Input: part model. Units: mm. Frame: model coordinates. Face numbers are marked on the shaded views. A direction names the side the tool comes from. Coordinates: 2 decimals unless noted, no trailing zeros. Order: outer loops, then holes, each group sorted by start corner. A loop starts at its lowest first (then second) coordinate and runs counter-clockwise, first axis right, second up. Notation, with made-up numbers: (0, -8.75) - (46, -8.75) arc R20 ccw to (46, 3.25) - close; hole circle Ø2 at (29, 5.5). An arc over 180 degrees is marked (long way). Answer as CSV lines item,"result". Start each with the question number.
Item 1: Draft query along Y for the marked faces 1, 2 and 3. Return one class per face: +Y half, -Y half, draft (parallel to the pull), parting line (faces both ways), or undercut.
Item 2: First-contact query: pin 1 (6 mm diameter, centred on x = -12, y = 4.5, fed in from -Z); pin 2 (11 mm diameter, centred on x = -1.5, z = 37.5, fed in from +Y); pin 3 (1 mm diameter, centred on x = 11.5, z = 77, fed in from +Y). Flat tips, straight axial feed; report the tip coordinate or a pass-through.
Item 3: Section D-D (x = 17). Output: boundary loops of the cut face in (y, z), and give its area (3 significant figures).
Item 4: Access query for the marked faces 4 and 5. Directions: +Z, -Z, +X, -X, +Y, -Y. A direction counts if a zero-diameter tool reaches every point of the face in a straight line with its end or side. Return the directions, or none.
Item 5: Material intervals for line 1 along Z through (x, y) = (0, -14); line 2 along X through (y, z) = (3, 63.5); line 3 along Y through (x, z) = (-1, 41.5), sorted ascending.
Item 6: Section A-A (x = 0). Output: boundary loops of the cut face in (y, z), and give its area (3 significant figures).
Item 7: Section C-C (y = 8.5). Output: boundary loops of the cut face in (x, z), and give its area (3 significant figures).
Item 8: Section B-B (z = 83.5). Output: boundary loops of the cut face in (x, y) (1 decimal), and give its area (3 significant figures).
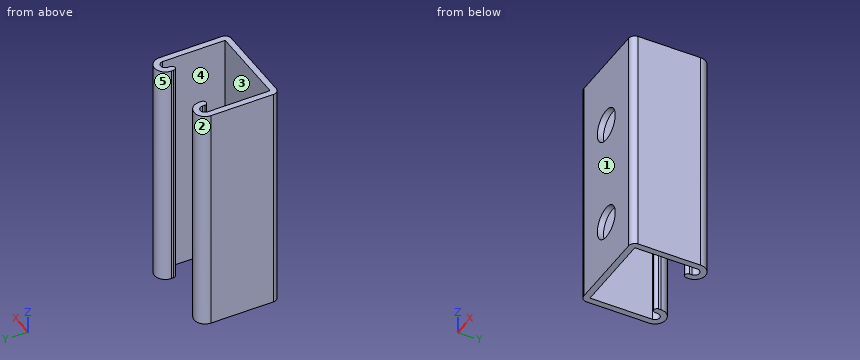
from build123d import *

# Parameters (mm, degrees)
BASE_EXTRUDE_DEPTH = 101.6
HOLE1_START        = -15.0114
HOLE1_OUTLINE_R    = 7.14375
HOLE1_DEPTH        = 2.6924
LPATTERN2_COUNT    = 2
LPATTERN2_PITCH    = 47.625


# Read off the part's stored shape, not the designer's step: Hole1
with BuildPart() as part:
    # Sketch1 → Base-Extrude (new body)
    with BuildSketch(Plane.XY):
        with BuildLine():
            Line((-20.6375, 15.1511), (-20.6375, -12.319))
            ThreePointArc((-20.6375, -12.319), (-19.848914298, -14.222814298), (-17.9451, -15.0114))
            Line((-17.9451, -15.0114), (17.9451, -15.0114))
            ThreePointArc((17.9451, -15.0114), (19.848914298, -14.222814298), (20.6375, -12.319))
            Line((20.6375, -12.319), (20.6375, 15.1511))
            ThreePointArc((20.6375, 15.1511), (15.875, 19.9136), (11.1125, 15.1511))
            Line((11.1125, 15.1511), (11.1125, 14.11605))
            ThreePointArc((11.1125, 14.11605), (12.4587, 12.76985), (13.8049, 14.11605))
            Line((13.8049, 14.11605), (13.8049, 15.1511))
            ThreePointArc((13.8049, 15.1511), (15.875, 17.2212), (17.9451, 15.1511))
            Line((17.9451, 15.1511), (17.9451, -12.319))
            Line((17.9451, -12.319), (-17.9451, -12.319))
            Line((-17.9451, -12.319), (-17.9451, 15.1511))
            ThreePointArc((-17.9451, 15.1511), (-15.875, 17.2212), (-13.8049, 15.1511))
            Line((-13.8049, 15.1511), (-13.8049, 14.11605))
            ThreePointArc((-13.8049, 14.11605), (-12.4587, 12.76985), (-11.1125, 14.11605))
            Line((-11.1125, 14.11605), (-11.1125, 15.1511))
            ThreePointArc((-11.1125, 15.1511), (-15.875, 19.9136), (-20.6375, 15.1511))
        make_face()
    extrude(amount=BASE_EXTRUDE_DEPTH)

    # Hole1 outline → Hole1 (cut)
    with BuildSketch(Plane(origin=(0, 0, 0), x_dir=(1, 0, 0), z_dir=(0, 1, 0)).offset(HOLE1_START)):
        with Locations((0, -23.8125)):
            Circle(HOLE1_OUTLINE_R)
    hole1 = extrude(amount=HOLE1_DEPTH, mode=Mode.SUBTRACT)

    # LPattern2: Hole1 ×2
    with Locations(*[(0, 0, i * LPATTERN2_PITCH) for i in range(1, LPATTERN2_COUNT)]):
        add(hole1, mode=Mode.SUBTRACT)


solid = part.part
Determined:
1,face 1,"-Y half"
1,face 2,"+Y half"
1,face 3,"undercut"
2,pin 1,"passes through"
2,pin 2,"stops at y = -12.32"
2,pin 3,"stops at y = 17.92"
3,outline,"(-15.01, 0) - (-12.32, 0) - (-12.32, 101.6) - (-15.01, 101.6) - close; (16.89, 0) - (19.78, 0) - (19.78, 101.6) - (16.89, 101.6) - close"
3,area,"567 mm^2"
4,face 4,"+Z, -Z"
4,face 5,"+Z, -Z, +Y"
5,line 1,"z = 0 to 16.67, 30.96 to 64.29, 78.58 to 101.6"
5,line 2,"x = -20.64 to -17.95, 17.95 to 20.64"
5,line 3,"y = -15.01 to -12.32"
6,outline,"(-15.01, 0) - (-12.32, 0) - (-12.32, 16.67) - (-15.01, 16.67) - close; (-15.01, 30.96) - (-12.32, 30.96) - (-12.32, 64.29) - (-15.01, 64.29) - close; (-15.01, 78.58) - (-12.32, 78.58) - (-12.32, 101.6) - (-15.01, 101.6) - close"
6,area,"197 mm^2"
7,outline,"(-20.64, 0) - (-17.95, 0) - (-17.95, 101.6) - (-20.64, 101.6) - close; (17.95, 0) - (20.64, 0) - (20.64, 101.6) - (17.95, 101.6) - close"
7,area,"547 mm^2"
8,outline,"(-20.6, -12.3) arc R2.7 ccw to (-17.9, -15) - (17.9, -15) arc R2.7 ccw to (20.6, -12.3) - (20.6, 15.2) arc R4.8 ccw to (11.1, 15.2) - (11.1, 14.1) arc R1.3 ccw to (13.8, 14.1) - (13.8, 15.2) arc R2.1 cw to (17.9, 15.2) - (17.9, -12.3) - (-17.9, -12.3) - (-17.9, 15.2) arc R2.1 cw to (-13.8, 15.2) - (-13.8, 14.1) arc R1.3 ccw to (-11.1, 14.1) - (-11.1, 15.2) arc R4.8 ccw to (-20.6, 15.2) - close"
8,area,"325 mm^2"
